Here's the drawing with two shaded views (mm, measured from the low corner). I have some questions. Give positions to 0.01 mm unless a question says otherwise; leave off trailing zeros. Write each loop counter-clockwise with the first axis right and the second up, starting at its lowest first coordinate (ties: lowest second). Pieces come first, ordered by that corner, then holes. Notation, with made-up numbers: M 68.25,32 L 125.25,32 A14 cw 125.25,36 Z; hole C 48.25,-9 d6. An arc over 180 degrees is marked long. Answer as a JSON object with one key per item and string values. Group by question number.
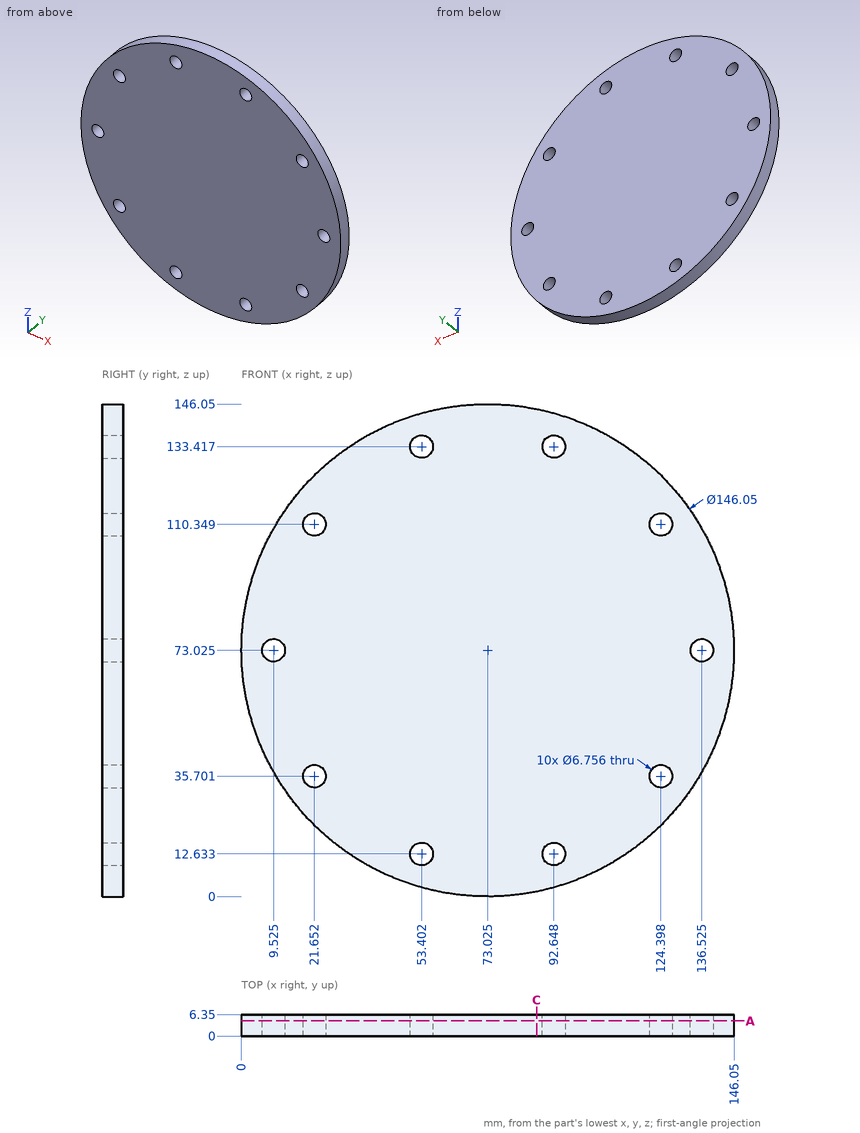
1) If we section it at A-A, the plane y = 4.5: Give the number of separate pieces and of enclosed holes in the cut face, plus the area to 3 significant figures.
2) Please list where these lines run through material, in increasing order: line 1 along Z through (x, y) = (92, 3); line 2 along Z through (x, y) = (124, 4.5) (1 decimal); line 3 along X through (y, z) = (4.75, 34) (1 decimal). Write a range as from..to.
3) I'm going to push flat-ended pins straight in: pin 1 (1 mm diameter, centred on y = 2, z = 57, fed in from -X); pin 2 (1.5 mm diameter, centred on y = 4.5, z = 75.5, fed in from +X). Where does each tip first touch, or does it pass through?
4) If we section it at C-C, the plane x = 87.5: List the corners of the cut face in (y, z) for me.
Taken from the geometry:
{
 "1": {"separate pieces": "1", "enclosed holes": "10", "area": "16,400 mm²"},
 "2": {"line 1": "2.51..9.32, 15.95..130.1, 136.73..143.54", "line 2": "20.7..32.3, 39.1..107, 113.7..125.3", "line 3": "11.3..18.7, 24.6..121.5, 127.3..134.7"},
 "3": {"pin 1": "x = 1.67", "pin 2": "x = 146.03"},
 "4": {"outline": "M 0,1.45 L 6.35,1.45 L 6.35,144.6 L 0,144.6 Z"}
}
